Could you check a few things on this model? Use its own coordinates, in mm. A direction names the side the tool comes from. Give positions to 0.01 mm unless a question says otherwise; leave off trailing zeros. Loops run counter-clockwise (first coordinate to the right, second up) from the corner with the lowest first, then second, coordinate; pieces in that order, holes last. Notation, with made-up numbers: (-22, 84.5) - (35, 84.5) arc R20 cw to (35, 111.5) - close; hole circle Ø4 at (1, 31). An arc over 180 degrees is marked (long way). One line per item, written item: value. Start each with the question number.
Q1. I want a section at B-B (z = 69.5). Please give me the cut outline in (x, y), then the cut area to 3 significant figures.
Q2. I want a section at D-D (x = 4.75). Please give me the cut outline in (y, z).
Q3. If we mould it in two halves opening along Y, with no side actions, what happens to faces 5 (the face through (7, -25, 0)), 6 (the face through (-0.53, 29.41, 66.41)), 7 (the face through (0, 30, 1))? For each: released by +Y, released by -Y, zero draft, split by the parting line, or undercut.
Q4. If I drill on line 1 (Y direction, x = -7.15, z = -80) (3 decimals); line 2 (X direction, y = -10.5, z = 75.5); line 3 (Y direction, x = 2.25, z = 35.5), over which ranges is the centre line in solid material (lowest first)? Write a range as from..to.
Q5. I'm going to push flat-ended pins straight in: P1, Ø6, axis at x = -2.5, y = -15.5, coming from the -Z side; P2, Ø3, axis at x = 0, z = -79, coming from the -Y side; P3, Ø2.5, axis at y = 0, z = -80, coming from the -X side. Where does each tip first touch, or does it pass through?
Q6. I want a section at C-C (y = 9). Please give me the cut outline in (x, z).
Q7. For faces 1 (the face through (0, -28.8, 1)), 2 (the face through (0.63, 29.41, -66.41)), 3 (the face through (0, -29, -59)), 4 (the face through (-6.9, -0.6, 78.6)), which set-ups out of +Z, -Z, +X, -X, +Y, -Y let a thin tool reach every point of the face, with its end or its side?
Q8. I want a section at A-A (z = 0). Please give me the cut outline in (x, y) (3 decimals).
```python
from build123d import *

# Parameters (mm, degrees)
SKETCH_1_W          = 15
SKETCH_1_H          = 60
SKETCH_1_W_2        = 12.6
SKETCH_1_H_2        = 57.6
EXTRUDE_1_DEPTH     = 85
SKETCH_2_R          = 2
CUT_EXTRUDE_1_DEPTH = 10
SKETCH_3_R          = 1.525
CUT_EXTRUDE_2_DEPTH = 10
SKETCH_4_R          = 1.525
CUT_EXTRUDE_3_DEPTH = 10
CUT_EXTRUDE_4_DEPTH = 10


with BuildPart() as part:
    # 草图1 → 凸台-拉伸1 (new, symmetric)
    with BuildSketch(Plane.XY):
        Rectangle(SKETCH_1_W, SKETCH_1_H)
        Rectangle(SKETCH_1_W_2, SKETCH_1_H_2, mode=Mode.SUBTRACT)
    extrude(amount=EXTRUDE_1_DEPTH, both=True)

    # 草图2 → 切除-拉伸1 (cut)
    with BuildSketch(Plane(origin=(0, -28.8, 0), x_dir=(1, 0, 0), z_dir=(0, 1, 0))):
        with Locations(Location((0, -79, 0), (0, 0, 270))):
            Circle(SKETCH_2_R)
        with Locations(Location((0, -61, 0), (0, 0, 270))):
            Circle(SKETCH_2_R)
    cut_extrude_1 = extrude(amount=-CUT_EXTRUDE_1_DEPTH, mode=Mode.SUBTRACT)

    # 镜向1: 切除-拉伸1 across plane
    add(cut_extrude_1.mirror(Plane.XY), mode=Mode.SUBTRACT)

    # 草图3 → 切除-拉伸2 (cut)
    with BuildSketch(Plane(origin=(0, 30, 0), x_dir=(1, 0, 0), z_dir=(0, 1, 0))):
        with Locations(Location((0.05, -75, 0), (0, 0, 270))):
            Circle(SKETCH_3_R)
        with Locations(Location((0.05, -65, 0), (0, 0, 270))):
            Circle(SKETCH_3_R)
        with Locations(Location((0.05, 65, 0), (0, 0, 90))):
            Circle(SKETCH_3_R)
        with Locations(Location((0.05, 75, 0), (0, 0, 90))):
            Circle(SKETCH_3_R)
    extrude(amount=-CUT_EXTRUDE_2_DEPTH, mode=Mode.SUBTRACT)

    # 草图4 → 切除-拉伸3 (cut)
    with BuildSketch(Plane(origin=(-6.3, 0, 0), x_dir=(0, 0, -1), z_dir=(1, 0, 0))):
        with Locations((0, -20)):
            Circle(SKETCH_4_R)
        Circle(SKETCH_4_R)
        with Locations((0, 20)):
            Circle(SKETCH_4_R)
        with Locations((-80, -20)):
            Circle(SKETCH_4_R)
        with Locations((-80, 0)):
            Circle(SKETCH_4_R)
        with Locations((-80, 20)):
            Circle(SKETCH_4_R)
        with Locations(Location((80, 20, 0), (0, 0, 90))):
            Circle(SKETCH_4_R)
        with Locations(Location((80, 0, 0), (0, 0, 90))):
            Circle(SKETCH_4_R)
        with Locations(Location((80, -20, 0), (0, 0, 90))):
            Circle(SKETCH_4_R)
    extrude(amount=-CUT_EXTRUDE_3_DEPTH, mode=Mode.SUBTRACT)

    # 草图5 → 切除-拉伸4 (cut)
    with BuildSketch(Plane(origin=(7.5, 0, 0), x_dir=(0, 0, -1), z_dir=(1, 0, 0))):
        with BuildLine():
            Line((-5, -20), (-5, 20))
            ThreePointArc((-5, 20), (0, 25), (5, 20))
            Line((5, 20), (5, -20))
            ThreePointArc((5, -20), (0, -25), (-5, -20))
        make_face()
    extrude(amount=-CUT_EXTRUDE_4_DEPTH, mode=Mode.SUBTRACT)


solid = part.part
```
Worked answers:
1. outline: (-7.5, -30) - (7.5, -30) - (7.5, 30) - (-7.5, 30) - close; hole (-6.3, -28.8) - (6.3, -28.8) - (6.3, 28.8) - (-6.3, 28.8) - close
1. area: 174 mm²
2. outline: (-30, -85) - (-28.8, -85) - (-28.8, 85) - (-30, 85) - close; (28.8, -85) - (30, -85) - (30, 85) - (28.8, 85) - close
3. face 5: undercut
3. face 6: zero draft
3. face 7: released by +Y
4. line 1: y = -30..-21.525, -18.475..-1.525, 1.525..18.475, 21.525..30
4. line 2: x = -7.5..-6.3, 6.3..7.5
4. line 3: y = -30..-28.8, 28.8..30
5. P1: passes through
5. P2: stops at y = 28.8
5. P3: stops at x = 6.3
6. outline: (-7.5, -85) - (-6.3, -85) - (-6.3, 85) - (-7.5, 85) - close; (6.3, -85) - (7.5, -85) - (7.5, -5) - (6.3, -5) - close; (6.3, 5) - (7.5, 5) - (7.5, 85) - (6.3, 85) - close
7. face 1: +Z, -Z
7. face 2: +Y
7. face 3: -Y
7. face 4: -X
8. outline: (-7.5, -30) - (7.5, -30) - (7.5, -25) - (6.3, -25) - (6.3, -28.8) - (-6.3, -28.8) - (-6.3, -21.525) - (-7.5, -21.525) - close; (-7.5, -18.475) - (-6.3, -18.475) - (-6.3, -1.525) - (-7.5, -1.525) - close; (-7.5, 1.525) - (-6.3, 1.525) - (-6.3, 18.475) - (-7.5, 18.475) - close; (-7.5, 21.525) - (-6.3, 21.525) - (-6.3, 28.8) - (6.3, 28.8) - (6.3, 25) - (7.5, 25) - (7.5, 30) - (-7.5, 30) - close
